Model file for the job. Use its own axes, mm. Give positions to 0.01 mm unless a question says otherwise; leave off trailing zeros. Loops run counter-clockwise (first coordinate to the right, second up) from the corner with the lowest first, then second, coordinate; pieces in that order, holes last. Notation, with made-up numbers: M -19.75,-11 L -12.75,-11 A6 cw -12.75,-6 Z; hole C 20.5,-34.5 d9. An arc over 180 degrees is marked long. Answer in a Markdown table with one row per item.
```python
from build123d import *

# Parameters (mm, degrees)
ESQUISSE2_R        = 1.5
ESQUISSE2_R_2      = 3
ESQUISSE2_R_3      = 8.25
ESQUISSE2_W        = 5
ESQUISSE2_H        = 10
BOSS_EXTRU_1_DEPTH = 3


with BuildPart() as part:
    # Esquisse2 → Boss.-Extru.1 (new body)
    with BuildSketch(Plane.XY):
        Polygon((-71.711544081, -86.276689775), (-71.711544081, -71.276689775), (-74.711544081, -71.276689775), (-74.711544081, -61.276689775), (-71.711544081, -61.276689775), (-71.711544081, -46.276689775), (-74.711544081, -46.276689775), (-74.711544081, -36.276689775), (-71.711544081, -36.276689775), (-71.711544081, -21.276689775), (-74.711544081, -21.276689775), (-74.711544081, -11.276689775), (-71.711544081, -11.276689775), (-71.711544081, 3.970120669), (-74.711544081, 3.970120669), (-74.711544081, 13.970120669), (-71.711544081, 13.970120669), (-71.711544081, 28.970120669), (-74.711544081, 28.970120669), (-74.711544081, 38.970120669), (-71.711544081, 38.970120669), (-71.711544081, 53.970120669), (-91.711544081, 53.970120669), (-91.711544081, 92.970120669), (-81.711544081, 92.970120669), (-81.711544081, 89.970120669), (-71.711544081, 89.970120669), (-71.711544081, 92.970120669), (-61.711544081, 92.970120669), (-61.711544081, 89.970120669), (-51.711544081, 89.970120669), (-51.711544081, 92.970120669), (-41.711544081, 92.970120669), (-41.711544081, 89.970120669), (-31.711544081, 89.970120669), (-31.711544081, 92.970120669), (-21.711544081, 92.970120669), (-21.711544081, 88.970120669), (-18.711544081, 88.970120669), (-18.711544081, 78.970120669), (-21.711544081, 78.970120669), (-21.711544081, 63.970120669), (-18.711544081, 63.970120669), (-18.711544081, 53.970120669), (-21.711544081, 53.970120669), (-21.711544081, 38.970120669), (-18.711544081, 38.970120669), (-18.711544081, 28.970120669), (-21.711544081, 28.970120669), (-21.711544081, 13.970120669), (-18.711544081, 13.970120669), (-18.711544081, 3.970120669), (-21.711544081, 3.970120669), (-21.711544081, -11.276689775), (-18.711544081, -11.276689775), (-18.711544081, -21.276689775), (-21.711544081, -21.276689775), (-21.711544081, -36.276689775), (-18.711544081, -36.276689775), (-18.711544081, -46.276689775), (-21.711544081, -46.276689775), (-21.711544081, -61.276689775), (-18.711544081, -61.276689775), (-18.711544081, -71.276689775), (-21.711544081, -71.276689775), (-21.711544081, -86.276689775), align=None)
        with Locations((-42.211544081, -51.276689775)):
            Circle(ESQUISSE2_R, mode=Mode.SUBTRACT)
        with Locations((-24.211544081, -51.276689775)):
            Circle(ESQUISSE2_R, mode=Mode.SUBTRACT)
        with Locations(Location((-33.211544081, 42.823310225, 0), (0, 0, 180))):
            Circle(ESQUISSE2_R_2, mode=Mode.SUBTRACT)
        with Locations(Location((-42.211544081, 22.223310225, 0), (0, 0, 180))):
            Circle(ESQUISSE2_R, mode=Mode.SUBTRACT)
        with Locations(Location((-24.211544081, 22.223310225, 0), (0, 0, 180))):
            Circle(ESQUISSE2_R, mode=Mode.SUBTRACT)
        with Locations((-80.711544081, 78.970120669)):
            Circle(ESQUISSE2_R_3, mode=Mode.SUBTRACT)
        with Locations((-54.211544081, 78.970120669)):
            Circle(ESQUISSE2_R_3, mode=Mode.SUBTRACT)
        with Locations((-33.211544081, -71.876689775)):
            Circle(ESQUISSE2_R_2, mode=Mode.SUBTRACT)
        with Locations((-33.078903677, -14.419560471)):
            Rectangle(ESQUISSE2_W, ESQUISSE2_H, mode=Mode.SUBTRACT)
    extrude(amount=BOSS_EXTRU_1_DEPTH)


solid = part.part
```
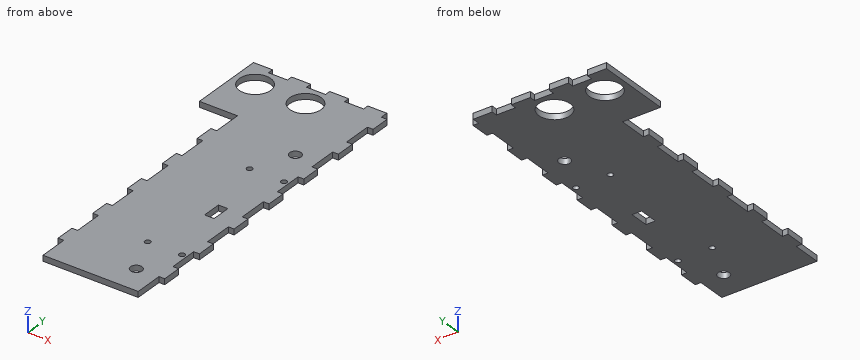
(1) Flat gauge pins, fed straight in: P1, Ø1.5, axis at y = -15, z = 2, coming from the -X side; P2, Ø1, axis at y = -25, z = 2.5, coming from the -X side; P3, Ø1.5, axis at x = -20.5, z = 1, coming from the -Y side. Where does each tip first touch, or does it go through?
Established:
| item | result |
|---|---|
| P1 | stops at x = -74.71 |
| P2 | stops at x = -71.71 |
| P3 | stops at y = -71.28 |
(2) Saw through at A-A, the plane x = -58.5. Give the cut face in (y, z).
Established:
| item | result |
|---|---|
| outline | M -86.28,0 L 71.92,0 L 71.92,3 L -86.28,3 Z; M 86.02,0 L 89.97,0 L 89.97,3 L 86.02,3 Z |
(3) Saw through at D-D, the plane z = 1.25. Count the separate pieces of the cut face and the enclosed holes in it, and give its area (3 significant figures).
Established:
| item | result |
|---|---|
| separate pieces | 1 |
| enclosed holes | 9 |
| area | 9,450 mm2 |
(4) Saw through at C-C, the plane y = 32. Give the cut face in (x, z), and give its area (3 significant figures).
Established:
| item | result |
|---|---|
| outline | M -74.71,0 L -18.71,0 L -18.71,3 L -74.71,3 Z |
| area | 168 mm2 |
(5) Wall check: L1, parallel to Y at x = -81, z = 0.55; L2, parallel to Y at x = -23, z = 0.45; L3, parallel to Y at x = -23.5, z = 1.2. Give the ranges that are in metal, low to high.
Established:
| item | result |
|---|---|
| L1 | y = 53.97 to 70.73, 87.22 to 89.97 |
| L2 | y = -86.28 to -52.16, -50.39 to 21.34, 23.11 to 92.97 |
| L3 | y = -86.28 to -52.6, -49.96 to 20.9, 23.54 to 92.97 |
(6) Saw through at B-B, the plane y = 77. Give the cut face in (x, z).
Established:
| item | result |
|---|---|
| outline | M -91.71,0 L -88.72,0 L -88.72,3 L -91.71,3 Z; M -72.7,0 L -62.22,0 L -62.22,3 L -72.7,3 Z; M -46.2,0 L -21.71,0 L -21.71,3 L -46.2,3 Z |
